The listing builds one solid part. Answer for the finished solid, in the listing's coordinates (mm). Face numbers are marked on the shaded views. A direction names the side the tool comes from. Coordinates: 2 decimals unless noted, no trailing zeros. Write each loop counter-clockwise with the first axis right and the second up, starting at its lowest first coordinate (ties: lowest second). Pieces come first, ordered by that corner, then holes.
from build123d import *

# Parameters (mm, degrees)
F0_W      = 15
F0_H      = 55
F1_DEPTH  = 15
F2_W      = 30
F2_H      = 55
F3_DEPTH  = 4
F4_W      = 4.9988695979
F4_H      = 5.0033593178
F5_DEPTH  = 25
F6_W      = 5.0042228401
F6_H      = 5.0039739907
F7_DEPTH  = 25
F8_R      = 5
F9_DEPTH  = 5
F10_R     = 5
F11_DEPTH = 5
F12_R     = 3
F13_DEPTH = 10
F14_R     = 2.9985824227
F15_DEPTH = 10
F16_R     = 10
F17_DEPTH = 2.5
F18_R     = 10
F19_DEPTH = 2.5
F20_R     = 10
F21_DEPTH = 2.5
F22_R     = 10
F23_DEPTH = 2.5
F24_R     = 2.5
F25_DEPTH = 2
F26_R     = 2.5
F27_DEPTH = 2
F28_R     = 2.5
F29_DEPTH = 2
F30_R     = 2.5
F31_DEPTH = 2


with BuildPart() as f1:
    # F0 (on Top) → F1 (new body)
    with BuildSketch(Plane.XY):
        Rectangle(F0_W, F0_H)
    extrude(amount=-F1_DEPTH)

    # F2 (on Top) → F3 (join)
    with BuildSketch(Plane.XY):
        Rectangle(F2_W, F2_H)
    extrude(amount=F3_DEPTH)

    # F4 (on Top) → F5 (cut)
    with BuildSketch(Plane.XY):
        with Locations((12.500565201, -24.9983203411)):
            Rectangle(F4_W, F4_H)
    extrude(amount=F5_DEPTH, mode=Mode.SUBTRACT)

    # F6 (on Top) → F7 (cut)
    with BuildSketch(Plane.XY):
        with Locations((12.49788858, 24.9980130047)):
            Rectangle(F6_W, F6_H)
    extrude(amount=F7_DEPTH, mode=Mode.SUBTRACT)

    # F8 (on face) → F9 (join)
    with BuildSketch(Plane.XZ.offset(27.5)):
        with Locations((0, -7.500606589)):
            Circle(F8_R)
    extrude(amount=F9_DEPTH)

    # F10 (on face) → F11 (join)
    with BuildSketch(Plane(origin=(0, 27.5, 0), x_dir=(-1, 0, 0), z_dir=(0, 1, 0))):
        with Locations((0, -7.5018298812)):
            Circle(F10_R)
    extrude(amount=F11_DEPTH)

    # F12 (on Right) → F13 (join, symmetric)
    with BuildSketch(Plane.YZ):
        with Locations((-14.9961104617, -11.996043846)):
            Circle(F12_R)
    extrude(amount=F13_DEPTH, both=True)

    # F14 (on Right) → F15 (join, symmetric)
    with BuildSketch(Plane.YZ):
        with Locations((15.0015540421, -12.0014175773)):
            Circle(F14_R)
    extrude(amount=F15_DEPTH, both=True)

    # F16 (on face) → F17 (join)
    with BuildSketch(Plane.YZ.offset(10)):
        with Locations((-14.9961104617, -11.996043846)):
            Circle(F16_R)
    extrude(amount=F17_DEPTH)

    # F18 (on face) → F19 (join)
    with BuildSketch(Plane.YZ.offset(10)):
        with Locations((15.0015540421, -12.0014175773)):
            Circle(F18_R)
    extrude(amount=F19_DEPTH)

    # F20 (on face) → F21 (join)
    with BuildSketch(Plane(origin=(-10, 0, 0), x_dir=(0, -1, 0), z_dir=(-1, 0, 0))):
        with Locations((-15.0015540421, -12.0014175773)):
            Circle(F20_R)
    extrude(amount=F21_DEPTH)

    # F22 (on face) → F23 (join)
    with BuildSketch(Plane(origin=(-10, 0, 0), x_dir=(0, -1, 0), z_dir=(-1, 0, 0))):
        with Locations((14.9961104617, -11.996043846)):
            Circle(F22_R)
    extrude(amount=F23_DEPTH)

    # F24 (on face) → F25 (join)
    with BuildSketch(Plane.YZ.offset(12.5)):
        with Locations((-14.9961104617, -11.996043846)):
            Circle(F24_R)
    extrude(amount=F25_DEPTH)

    # F26 (on face) → F27 (join)
    with BuildSketch(Plane.YZ.offset(12.5)):
        with Locations((15.0015540421, -12.0014175773)):
            Circle(F26_R)
    extrude(amount=F27_DEPTH)

    # F28 (on face) → F29 (join)
    with BuildSketch(Plane(origin=(-12.5, 0, 0), x_dir=(0, -1, 0), z_dir=(-1, 0, 0))):
        with Locations((14.9961104617, -11.996043846)):
            Circle(F28_R)
    extrude(amount=F29_DEPTH)

    # F30 (on face) → F31 (join)
    with BuildSketch(Plane(origin=(-12.5, 0, 0), x_dir=(0, -1, 0), z_dir=(-1, 0, 0))):
        with Locations((-15.0015540421, -12.0014175773)):
            Circle(F30_R)
    extrude(amount=F31_DEPTH)

    # F32 (on face) → F33 (revolve)
    with BuildSketch(Plane(origin=(0, 32.5, 0), x_dir=(-1, 0, 0), z_dir=(0, 1, 0))):
        with BuildLine():
            Line((0, -2.5018298812), (0, -12.5018298812))
            ThreePointArc((0, -12.5018298812), (5, -7.5018298812), (0, -2.5018298812))
        make_face()
    revolve(axis=Axis((0, 32.5, -7.5018298812), (0, 0, -1)))

    # F34 (on face) → F35 (revolve)
    with BuildSketch(Plane.XZ.offset(32.5)):
        with BuildLine():
            Line((0, -2.500606589), (0, -12.500606589))
            ThreePointArc((0, -12.500606589), (5, -7.500606589), (0, -2.500606589))
        make_face()
    revolve(axis=Axis((0, -32.5, -7.500606589), (0, 0, -1)))


solid = f1.part
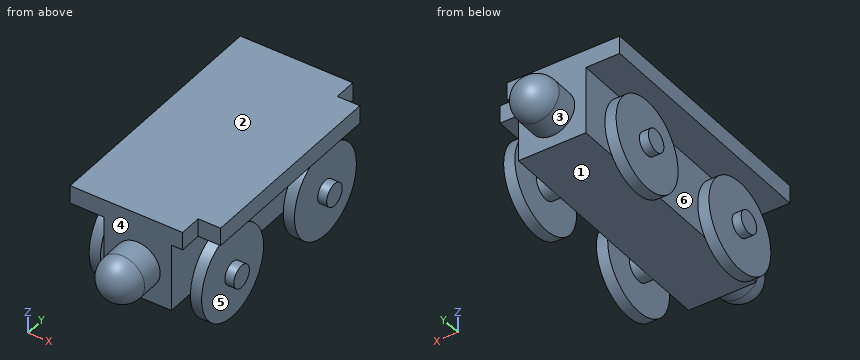
1. Section B-B on x = 0 is taken. Give the vertices of the cut face in (y, z), then the cut area to 3 significant figures.
Results found:
outline: (-32.5, -12.5) - (-27.5, -12.5) - (-27.5, -15) - (27.5, -15) - (27.5, -12.5) - (32.5, -12.5) arc R5 ccw to (32.5, -2.5) - (27.5, -2.5) - (27.5, 4) - (-27.5, 4) - (-27.5, -2.5) - (-32.5, -2.5) arc R5 ccw to start
area: 1,220 mm2
2. A tool of negligible diameter and unlimited length cuts with its end or side. For the marked faces 4, 5 and 6, from which of +Z, -Z, +X, -X, +Y, -Y can it reach the whole face along a straight path? Write none if from no direction.
Results found:
face 4: -Y
face 5: +X
face 6: none
3. Section D-D on y = 0 is taken. Give the vertices of the cut face in (x, z).
Results found:
outline: (-15, 0) - (-7.5, 0) - (-7.5, -15) - (7.5, -15) - (7.5, 0) - (15, 0) - (15, 4) - (-15, 4) - close
4. Flat-ended cylindrical pins translate along their axes: P1, Ø2, axis at y = -3.5, z = -4.5, coming from the +X side; P2, Ø5, axis at x = -3, y = -28.5, coming from the -Z side; P3, Ø1, axis at y = -2, z = -15, coming from the -X side. Find the tip coordinate at first contact, or state that the pin passes through.
Results found:
P1: stops at x = 7.5
P2: stops at z = -15
P3: stops at x = -7.5
5. Find the intervals of material crossed by L1, parallel to X at y = -10, z = -4; L2, parallel to X at y = -20.5, z = -18; L3, parallel to Y at x = 4, z = 0, in increasing order.
Results found:
L1: x = -12.5 to -10, -7.5 to 7.5, 10 to 12.5
L2: x = -12.5 to -10, 10 to 12.5
L3: y = -27.5 to 27.5
6. Section A-A on z = -18.25 is taken. Give the vertices of the cut face in (x, y), then the cut area to 3 significant figures.
Results found:
outline: (-12.5, -22.8) - (-10, -22.8) - (-10, -7.19) - (-12.5, -7.19) - close; (-12.5, 7.19) - (-10, 7.19) - (-10, 22.81) - (-12.5, 22.81) - close; (10, -22.8) - (12.5, -22.8) - (12.5, -7.19) - (10, -7.19) - close; (10, 7.19) - (12.5, 7.19) - (12.5, 22.81) - (10, 22.81) - close
area: 156 mm2
7. For a pull along X with two mould halves and no side action, classify the marked faces 1, 2 and 3 as pulls with the +X half, pulls with the -X half, needs draft (parallel to the pull), parting line crosses it, or undercut.
Results found:
face 1: undercut
face 2: needs draft
face 3: parting line crosses it
8. Section C-C on z = -3.5 is taken. Give the vertices of the cut face in (x, y).
Results found:
outline: (-12.5, -20.27) - (-10, -20.27) - (-10, -9.72) - (-12.5, -9.72) - close; (-12.5, 9.74) - (-10, 9.74) - (-10, 20.27) - (-12.5, 20.27) - close; (-7.5, -27.5) - (-3, -27.5) - (-3, -32.5) arc R3 ccw to (3, -32.5) - (3, -27.5) - (7.5, -27.5) - (7.5, 27.5) - (3, 27.5) - (3, 32.5) arc R3 ccw to (-3, 32.5) - (-3, 27.5) - (-7.5, 27.5) - close; (10, -20.27) - (12.5, -20.27) - (12.5, -9.72) - (10, -9.72) - close; (10, 9.74) - (12.5, 9.74) - (12.5, 20.27) - (10, 20.27) - close
